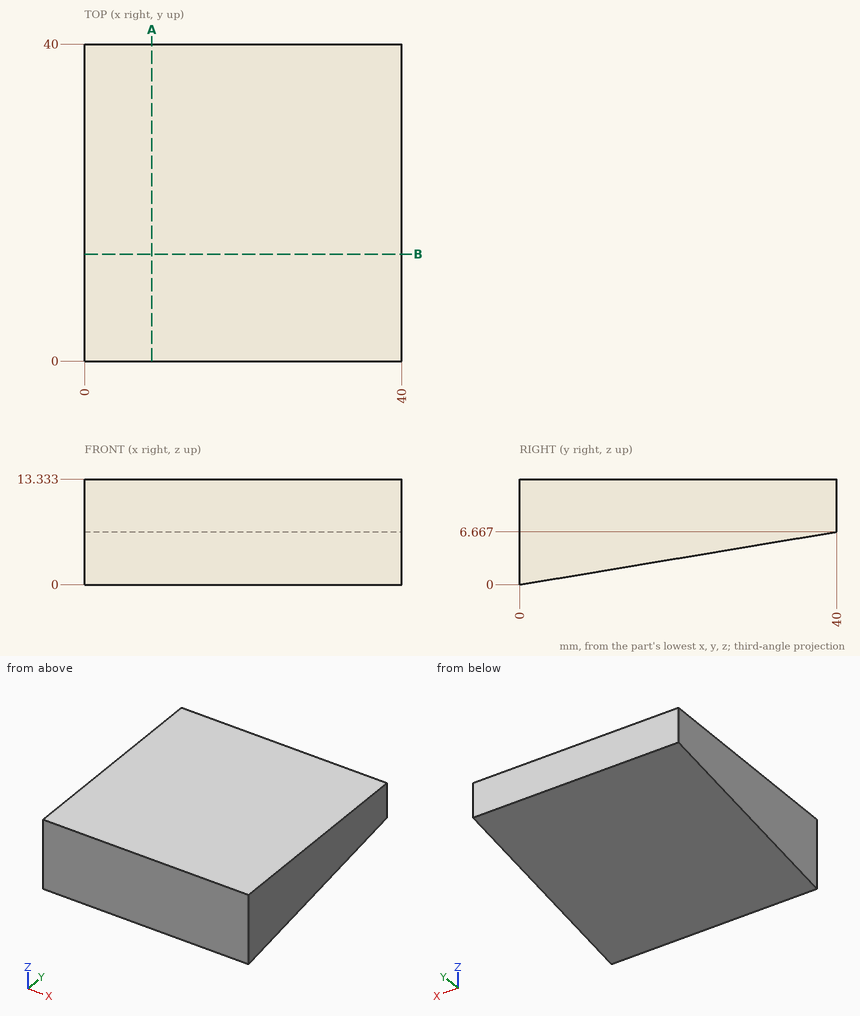
Job drawing, mm, ordinate dimensions from the low corner. One solid piece. Give positions to 0.01 mm unless a question says otherwise; leave off trailing zeros. Order: outer loops, then holes, each group sorted by start corner. A loop starts at its lowest first (then second) coordinate and runs counter-clockwise, first axis right, second up. Notation, with made-up numbers: M 75.25,-9 L 86.25,-9 A25 ccw 86.25,4 Z; hole C -37.75,80 d2. An arc over 180 degrees is marked long. Put each result on its own line as item: value. Start each with the question number.
(1) Band-saw the part on A-A on x = 8.5. Give the cut face in (y, z).
(2) Pin check, flat tips, straight feed: pin 1 Ø12 at (x, y) = (19.5, 9.5) entering from -Z; pin 2 Ø1 at (x, y) = (29, 18) entering from -Z. Stop position of each tip, or through.
(3) Drill centre lines: L1, parallel to Z at x = 19, y = 28; L2, parallel to Z at x = 22.5, y = 6.5. Where is each one in solid material? Low to high. Write a range as [from, to].
(4) Band-saw the part on B-B on y = 13.5. Give the cut face in (x, z).
Results below:
1. outline: M 0,0 L 40,6.67 L 40,13.33 L 0,13.33 Z
2. pin 1: stops at z = 0.58
2. pin 2: stops at z = 2.92
3. L1: z = [4.67, 13.33]
3. L2: z = [1.08, 13.33]
4. outline: M 0,2.25 L 40,2.25 L 40,13.33 L 0,13.33 Z
